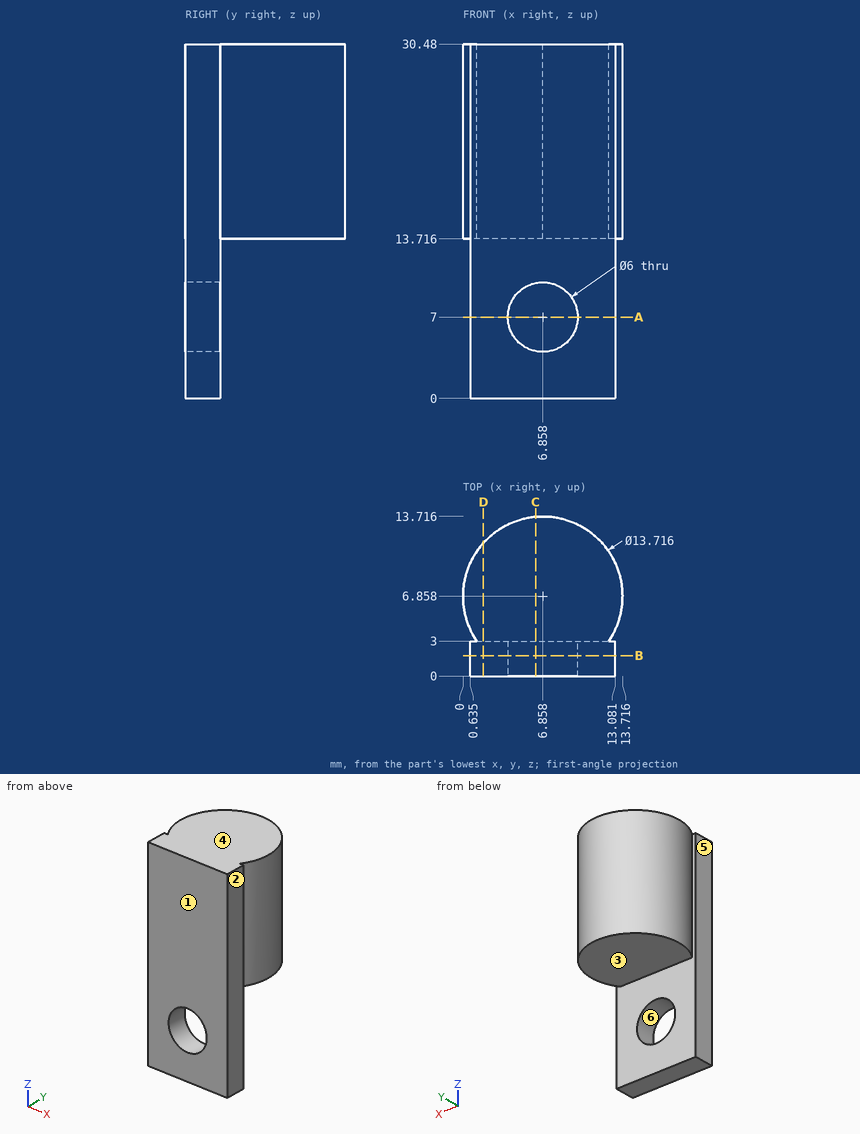
Geometry: see drawing. Coordinates: mm, zero at the bounding-box minimum. A direction names the side the tool comes from. Give positions to 0.01 mm unless a question says otherwise; leave off trailing zeros. Write each loop counter-clockwise with the first axis right and the second up, starting at its lowest first coordinate (ties: lowest second). Pieces come first, ordered by that corner, then holes. Notation, with made-up numbers: (15.25, 47) - (58.25, 47) arc R15 ccw to (58.25, 62) - close; hole circle Ø4 at (60.5, 44.25). An arc over 180 degrees is marked (long way). Return JSON: item names as keys, results as strings. Group by question number.
1) First-contact query: P1, Ø6, axis at y = 5, z = 21.5, coming from the +X side; P2, Ø5.5, axis at x = 7, y = 7, coming from the -Z side; P3, Ø0.9, axis at y = 2, z = 15.5, coming from the -X side (3 decimals); P4, Ø3, axis at x = 11.5, z = 7, coming from the +Y side. Flat tips, straight axial feed; report the tip coordinate or a pass-through.
2) Section A-A on z = 7. Return the cut outline in (x, y) (3 decimals).
3) Mould query, pull axis X, two halves, no side actions, for the marked faces 4, 5 and 6. Classes: released by +X, released by -X, zero draft, split by the parting line, or undercut.
4) Line query: line 1 (X direction, y = 0.8, z = 7) (3 decimals); line 2 (Y direction, x = 10, z = 2.5); line 3 (Z direction, x = 1.25, y = 5.5). Output: solid intervals per line, ascending.
5) Section C-C on x = 6.25. Return the cut outline in (y, z), plus the area to 3 significant figures.
6) Set-up query: the marked faces 1, 2 and 3. Return all of +Z, -Z, +X, -X, +Y, -Y with unobstructed straight access to the full face (end or side cutting, diameter ignored); none if empty.
7) Section D-D on x = 1.75. Return the cut outline in (y, z), plus the area to 3 significant figures.
8) Section B-B on y = 1.75. Return the cut outline in (x, z) (3 decimals).
Filled in:
{
 "1": {"P1": "stops at x = 13.72", "P2": "stops at z = 13.72", "P3": "stops at x = 0.635", "P4": "stops at y = 3"},
 "2": {"outline": "(0.635, 0) - (3.858, 0) - (3.858, 3) - (0.635, 3) - close; (9.858, 0) - (13.081, 0) - (13.081, 3) - (9.858, 3) - close"},
 "3": {"face 4": "zero draft", "face 5": "released by -X", "face 6": "undercut"},
 "4": {"line 1": "x = 0.635 to 3.858, 9.858 to 13.081", "line 2": "y = 0 to 3", "line 3": "z = 13.72 to 30.48"},
 "5": {"outline": "(0, 0) - (3, 0) - (3, 4.06) - (0, 4.06) - close; (0, 9.94) - (3, 9.94) - (3, 13.72) - (13.69, 13.72) - (13.69, 30.48) - (0, 30.48) - close", "area": "253 mm^2"},
 "6": {"face 1": "+Z, -Z, +X, -X, -Y", "face 2": "+Z, -Z, +X, -Y", "face 3": "-Z, +X, -X, +Y"},
 "7": {"outline": "(0, 0) - (3, 0) - (3, 13.72) - (11.43, 13.72) - (11.43, 30.48) - (0, 30.48) - close", "area": "233 mm^2"},
 "8": {"outline": "(0.635, 0) - (13.081, 0) - (13.081, 30.48) - (0.635, 30.48) - close; hole circle Ø6 at (6.858, 7)"}
}
